The listing builds one solid part. Answer for the finished solid, in the listing's coordinates (mm). Face numbers are marked on the shaded views. A direction names the side the tool comes from. Round coordinates to 2 decimals unless told otherwise and drop trailing zeros. Order: outer loops, then holes, each group sorted by start corner. A loop starts at its lowest first (then second) coordinate and runs counter-clockwise, first axis right, second up. Notation, with made-up numbers: (86.25, 18.25) - (128.25, 18.25) arc R28 ccw to (128.25, 55.25) - close; hole circle Ø9 at (33, -29.5). An arc over 180 degrees is marked (long way). Use CSV: the item, a comma, the result in double quotes. Start each with the question number.
Item 1: For the marked faces 4 and 5, determine the directions among +Z, -Z, +X, -X, +Y, -Y from which every point of the face is accessible in a straight line to the end or side of a thin tool.
Item 2: Flat-ended cylindrical pins translate along their axes: P1, Ø10.5, axis at x = -128.5, z = -81.5, coming from the +Y side; P2, Ø9.5, axis at x = 130, z = 80, coming from the +Y side. Find the tip coordinate at first contact, or state that the pin passes through.
Item 3: Find section C-C, the plane x = -11.5. Give the vertices of the cut face in (y, z).
Item 4: Determine the mould class of the marked faces 1, 2 and 3 for opening direction X: +X half, -X half, draft (parallel to the pull), parting line (faces both ways), or undercut.
Item 5: Find section A-A, the plane x = -130. Give the vertices of the cut face in (y, z), plus the area to 3 significant figures.
Item 6: Straight lines are drawn through the part: line 1 along Z through (x, y) = (130, 42); line 2 along Z through (x, y) = (-130, 8); line 3 along Z through (x, y) = (-68, 29.5). For each, find the intervals that lie inside material, in ascending order. Write a range as [from, to].
Item 7: Find section D-D, the plane y = 12. Give the vertices of the cut face in (x, z).
Item 8: Find section B-B, the plane z = 34.5. Give the vertices of the cut face in (x, y), plus the area to 3 significant figures.
```python
from build123d import *

# Parameters (mm, degrees)
CROQUIS1_W                   = 300
CROQUIS1_H                   = 200
SALIENTE_EXTRUIR1_DEPTH      = 50
TALADRO1_D                   = 12
TALADRO1_DEPTH               = 50.801082666
TALADRO1_CBORE_D             = 21
TALADRO1_CBORE_DEPTH         = 12
SIMETR_A2_COPY_1_D           = 12
SIMETR_A2_COPY_1_DEPTH       = 50.801082666
SIMETR_A2_COPY_1_CBORE_D     = 21
SIMETR_A2_COPY_1_CBORE_DEPTH = 12
CORTAR_EXTRUIR1_DEPTH        = 25
CORTAR_EXTRUIR2_DEPTH        = 51


with BuildPart() as part:
    # Croquis1 → Saliente-Extruir1 (new body)
    with BuildSketch(Plane(origin=(0, 0, 0), x_dir=(1, 0, 0), z_dir=(0, 1, 0))):
        Rectangle(CROQUIS1_W, CROQUIS1_H)
    extrude(amount=SALIENTE_EXTRUIR1_DEPTH)

    # Taladro1
    with Locations(Plane(origin=(0, 50, 0), x_dir=(1, 0, 0), z_dir=(0, 1, 0))):
        with Locations((-130, 80)):
            taladro1 = CounterBoreHole(TALADRO1_D / 2, TALADRO1_CBORE_D / 2, TALADRO1_CBORE_DEPTH, depth=TALADRO1_DEPTH)

    # Simetr_a1: Taladro1 across plane
    add(taladro1.mirror(Plane(origin=(0, 0, 0), x_dir=(0, 0, 1), z_dir=(1, 0, 0))), mode=Mode.SUBTRACT)

    # Simetr_a2: Taladro1 across plane
    add(taladro1.mirror(Plane.XY), mode=Mode.SUBTRACT)

    # Simetr_a2 copy 1
    with Locations(Plane(origin=(0, 50, 0), x_dir=(-1, 0, 0), z_dir=(0, 1, 0))):
        with Locations((-130, 80)):
            CounterBoreHole(SIMETR_A2_COPY_1_D / 2, SIMETR_A2_COPY_1_CBORE_D / 2, SIMETR_A2_COPY_1_CBORE_DEPTH, depth=SIMETR_A2_COPY_1_DEPTH)

    # Croquis4 → Cortar-Extruir1 (cut)
    with BuildSketch(Plane(origin=(0, 50, 0), x_dir=(1, 0, 0), z_dir=(0, 1, 0))):
        with BuildLine():
            Line((-75, 80), (75, 80))
            ThreePointArc((75, 80), (89.142135624, 74.142135624), (95, 60))
            Line((95, 60), (95, -60))
            ThreePointArc((95, -60), (89.142135624, -74.142135624), (75, -80))
            Line((75, -80), (-75, -80))
            ThreePointArc((-75, -80), (-89.142135624, -74.142135624), (-95, -60))
            Line((-95, -60), (-95, 60))
            ThreePointArc((-95, 60), (-89.142135624, 74.142135624), (-75, 80))
        make_face()
        with BuildLine():
            Line((-65, 65), (65, 65))
            ThreePointArc((65, 65), (72.071067812, 62.071067812), (75, 55))
            Line((75, 55), (75, -55))
            ThreePointArc((75, -55), (72.071067812, -62.071067812), (65, -65))
            Line((65, -65), (-65, -65))
            ThreePointArc((-65, -65), (-72.071067812, -62.071067812), (-75, -55))
            Line((-75, -55), (-75, 55))
            ThreePointArc((-75, 55), (-72.071067812, 62.071067812), (-65, 65))
        make_face(mode=Mode.SUBTRACT)
    extrude(amount=-CORTAR_EXTRUIR1_DEPTH, mode=Mode.SUBTRACT)

    # Croquis4_2 → Cortar-Extruir2 (cut)
    with BuildSketch(Plane(origin=(0, 50, 0), x_dir=(1, 0, 0), z_dir=(0, 1, 0))):
        with BuildLine():
            Line((-65, 65), (65, 65))
            ThreePointArc((65, 65), (72.071067812, 62.071067812), (75, 55))
            Line((75, 55), (75, -55))
            ThreePointArc((75, -55), (72.071067812, -62.071067812), (65, -65))
            Line((65, -65), (-65, -65))
            ThreePointArc((-65, -65), (-72.071067812, -62.071067812), (-75, -55))
            Line((-75, -55), (-75, 55))
            ThreePointArc((-75, 55), (-72.071067812, 62.071067812), (-65, 65))
        make_face()
    extrude(amount=-CORTAR_EXTRUIR2_DEPTH, mode=Mode.SUBTRACT)


solid = part.part
```
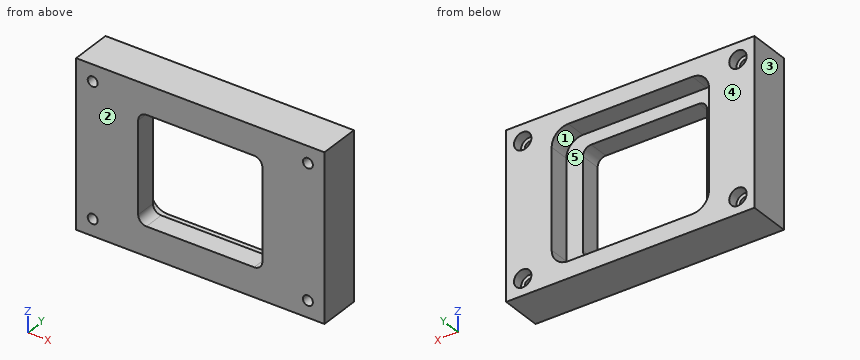
Worked out:
1,face 4,"+Z, -Z, +X, -X, +Y"
1,face 5,"+Y"
2,P1,"stops at y = 38"
2,P2,"passes through"
3,outline,"(0, -100) - (50, -100) - (50, -80) - (25, -80) - (25, -65) - (0, -65) - close; (0, 65) - (25, 65) - (25, 80) - (50, 80) - (50, 100) - (0, 100) - close"
4,face 1,"undercut"
4,face 2,"draft"
4,face 3,"-X half"
5,outline,"(0, -100) - (50, -100) - (50, -90.5) - (38, -90.5) - (38, -86) - (0, -86) - close; (0, -74) - (38, -74) - (38, -69.5) - (50, -69.5) - (50, 69.5) - (38, 69.5) - (38, 74) - (0, 74) - close; (0, 86) - (38, 86) - (38, 90.5) - (50, 90.5) - (50, 100) - (0, 100) - close"
5,area,"8,580 mm²"
6,line 1,"z = [-100, -90.5], [-69.5, 69.5], [90.5, 100]"
6,line 2,"z = [-100, -86], [-74, 74], [86, 100]"
6,line 3,"z = [-100, -80], [80, 100]"
7,outline,"(-150, -100) - (150, -100) - (150, 100) - (-150, 100) - close; hole circle Ø12 at (-130, -80); hole circle Ø12 at (-130, 80); hole (-75, -55) arc R10 ccw to (-65, -65) - (65, -65) arc R10 ccw to (75, -55) - (75, 55) arc R10 ccw to (65, 65) - (-65, 65) arc R10 ccw to (-75, 55) - close; hole circle Ø12 at (130, -80); hole circle Ø12 at (130, 80)"
8,outline,"(-150, 0) - (-75, 0) - (-75, 25) - (-95, 25) - (-95, 50) - (-150, 50) - close; (75, 0) - (150, 0) - (150, 50) - (95, 50) - (95, 25) - (75, 25) - close"
8,area,"6,500 mm²"
